Can you work these out from the model? Positions are in its coordinate system, mm. Coordinates: 2 decimals unless noted, no trailing zeros. Order: outer loops, then holes, each group sorted by start corner. A loop starts at its lowest first (then second) coordinate and runs counter-clockwise, first axis right, second up.
Autodesk Fusion 360 part; units mm, degrees
sketch "Sketch1" plane through (0, 0, 0) normal (0, 0, 1) x (1, 0, 0)
  circle A0 centre (0, 0) radius 24.5
  circle A1 centre (0, 0) radius 20
  dimension "d1" = 49
  dimension "d2" = 4.5
extrude "Extrude1" add sketch "Sketch1" along normal blind 300
ref_plane "WorkPlane1" through (0, 0, 10) normal (0, 0, 1) x (1, 0, 0)
ref_plane "WorkPlane2" through (0, 0, 300) normal (0, 0, 1) x (1, 0, 0)
ref_plane "WorkPlane3" through (0, 0, 242) normal (0, 0, 1) x (1, 0, 0)
sketch "Sketch2" plane through (0, 0, 0) normal (1, 0, 0) x (0, 0, -1)
  line L0 (-10, 42.4058) -> (-10, 1.4623) construction
  line L1 (-300, 66.3479) -> (-300, -66.3479) construction
  line L2 (-242, 79.6175) -> (-242, -79.6175) construction
  line L3 (-300, 0) -> (0, 0) construction
  line L4 (-10, 1.4623) -> (-10, 0) construction
  circle A0 centre (-10, 0) radius 4.25
  circle A1 centre (-242, 0) radius 6.5
  dimension "d8" = 8.5
  dimension "d9" = 13
extrude "Extrude2" cut sketch "Sketch2" along normal through all and the other way through all
1. Please list where these lines run through material, in increasing order: probe 1 along Z at (x, y) = (20.8, 0); probe 2 along Y at (x, z) = (0, 160.5); probe 3 along X at (y, z) = (-13, 179).
Completed:
probe 1: z = 0 to 5.75, 14.25 to 235.5, 248.5 to 300
probe 2: y = -24.5 to -20, 20 to 24.5
probe 3: x = -20.77 to -15.2, 15.2 to 20.77
2. Imagine slicing it at B-B on y = 9. Please give me the cut outline in (x, z).
Completed:
outline: (-22.79, 0) - (-17.86, 0) - (-17.86, 300) - (-22.79, 300) - close; (17.86, 0) - (22.79, 0) - (22.79, 300) - (17.86, 300) - close
3. Imagine slicing it at C-C on z = 195.5. Please give me the cut outline in (x, y).
Completed:
outline: circle Ø49 at (0, 0); hole circle Ø40 at (0, 0)
4. Imagine slicing it at A-A on x = 0. Please give me the cut outline in (y, z), then the cut area to 3 significant figures.
Completed:
outline: (-24.5, 0) - (-20, 0) - (-20, 300) - (-24.5, 300) - close; (20, 0) - (24.5, 0) - (24.5, 300) - (20, 300) - close
area: 2,700 mm2
5. Thinking about a two-plate mould opening in Y: for faces 1 (the cylindrical face through (19.076, -6.007, 147.9)), 2 (the cylindrical face through (23.37, -7.36, 147.9)), 3 (the flat face through (-9.2, -18, 0)), which applies, pulls with the +Y half, pulls with the -Y half, needs draft (parallel to the pull), parting line crosses it, or undercut?
Completed:
face 1: undercut
face 2: parting line crosses it
face 3: needs draft
6. I'm going to push flat-ended pins straight in: pin 1 (8 mm diameter, centred on x = 5, z = 265.5, fed in from +Y); pin 2 (10 mm diameter, centred on x = -16.5, z = 242, fed in from +Y); pin 3 (10 mm diameter, centred on x = 12, z = 266, fed in from +Y); pin 4 (7 mm diameter, centred on y = 0, z = 10, fed in from +X). Where does each tip first touch, or does it pass through?
Completed:
pin 1: stops at y = 24.48
pin 2: stops at y = 21.63
pin 3: stops at y = 23.48
pin 4: passes through
